Autodesk Inventor part; units mm, degrees
ref_plane "YZ Plane" through (0, 0, 0) normal (1, 0, 0) x (0, 1, 0)
ref_plane "XZ Plane" through (0, 0, 0) normal (0, 1, 0) x (-1, 0, 0)
ref_plane "XY Plane" through (0, 0, 0) normal (0, 0, 1) x (1, 0, 0)
sketch "Sketch4" plane through (0, 0, 0) normal (0, 1, 0) x (-1, 0, 0)
  line L0 (0.5, 0.5) -> (-0.5, 0.5)
  line L1 (-0.5, 0.5) -> (-0.5, -0.5)
  line L2 (-0.5, -0.5) -> (0.5, -0.5)
  line L3 (0.5, -0.5) -> (0.5, 0.5)
  line L4 (0.5, 0.5) -> (-0.5, -0.5) construction
  line L5 (-0.5, 0.5) -> (0.5, -0.5) construction
  point P0 (0, 0)
  dimension "d13" = 1
  dimension "d14" = 1
extrude "Extrusion4" add sketch "Sketch4" along normal blind 17.67
sketch "Sketch5" plane through (-0.5, 0, 0.5) normal (0, 0, 1) x (1, 0, 0)
  line L0 (1, 17.67) -> (0, 17.67)
  line L1 (1, 0) -> (1, 17.67)
  line L2 (0, 17.67) -> (1, 17.67)
  line L3 (1, 17.67) -> (1, 16.67)
  line L4 (1, 16.67) -> (0, 16.67)
  line L5 (0, 16.67) -> (0, 17.67)
  point P0 (0.5, 0)
  dimension "d17" = 1
extrude "Extrusion5" add sketch "Sketch5" along normal blind 3.1
properties part number "jst-vh-2p_wire"
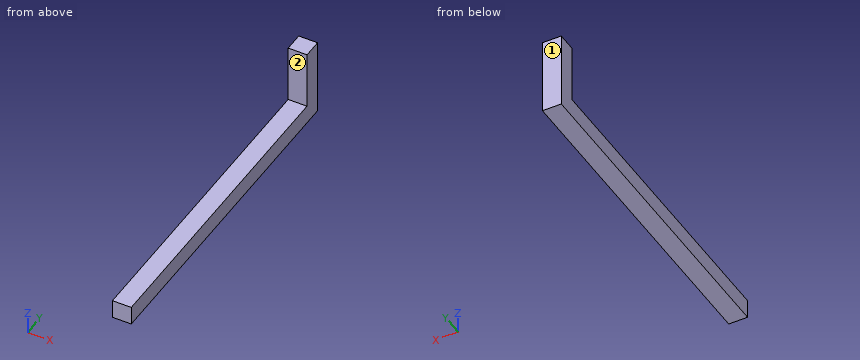
Verification items for the finished model (mm, model axes). Face numbers are marked on the shaded views. A direction names the side the tool comes from. Round coordinates to 2 decimals unless told otherwise and drop trailing zeros. Order: outer loops, then holes, each group sorted by start corner. A loop starts at its lowest first (then second) coordinate and runs counter-clockwise, first axis right, second up.
1. Section check A-A on x = 0.1. Record the cut outline in (y, z).
Final values:
outline: (0, -0.5) - (17.67, -0.5) - (17.67, 3.6) - (16.67, 3.6) - (16.67, 0.5) - (0, 0.5) - close
2. Section check C-C on z = 3.25. Record the cut outline in (x, y), then the cut area to 3 significant figures.
Final values:
outline: (-0.5, 16.67) - (0.5, 16.67) - (0.5, 17.67) - (-0.5, 17.67) - close
area: 1.00 mm2
3. Access from +Z, -Z, +X, -X, +Y, -Y to the whole of each face (thin tool, end or side, straight path). Record for the marked faces 1 and 2.
Final values:
face 1: +Z, -Z, +X, -X, +Y
face 2: +Z, +X, -X, -Y
4. Go/stop test with a flat-tipped pin: P1, Ø1.5, axis at y = 8.5, z = 2, coming from the -X side. Record where the tip stops, or that it passes through.
Final values:
P1: passes through
5. Section check B-B on y = 14.5. Record the cut outline in (x, z).
Final values:
outline: (-0.5, -0.5) - (0.5, -0.5) - (0.5, 0.5) - (-0.5, 0.5) - close
6. Thickness scan on L1, parallel to Y at x = 0.05, z = 2.2; L2, parallel to Z at x = 0, y = 15.5. Record the ranges inside material, lowest first.
Final values:
L1: y = 16.67 to 17.67
L2: z = -0.5 to 0.5
